Here's how the part is built. I have some questions about the finished solid (model axes, mm). Face numbers are marked on the shaded views. A direction names the side the tool comes from. Round coordinates to 2 decimals unless told otherwise and drop trailing zeros. Loops run counter-clockwise (first coordinate to the right, second up) from the corner with the lowest first, then second, coordinate; pieces in that order, holes last. Notation, with made-up numbers: (54.5, 60) - (99.5, 60) arc R18 ccw to (99.5, 72) - close; hole circle Ø1 at (46, 68.25). An arc over 180 degrees is marked (long way). Return JSON: item names as keys, results as strings. Group by question number.
```python
from build123d import *

# Parameters (mm, degrees)
F0_R     = 2.125
F1_DEPTH = 5
F3_DEPTH = 15
F4_R     = 2.125
F5_DEPTH = 5
F6_R     = 2.125
F7_DEPTH = 5
F9_DEPTH = 5
F10_SIZE = 10


with BuildPart() as f1:
    # F0 (on Top) → F1 (new body)
    with BuildSketch(Plane.XY):
        Polygon((0, 20), (0, 50), (-20, 50), (-20, 0), (30, 0), (30, 20), align=None)
        with Locations((-12.5, 7.5)):
            Circle(F0_R, mode=Mode.SUBTRACT)
        with Locations((20, 7.5)):
            Circle(F0_R, mode=Mode.SUBTRACT)
        with Locations((-12.5, 40)):
            Circle(F0_R, mode=Mode.SUBTRACT)
    extrude(amount=F1_DEPTH)

    # F2 (on face) → F3 (join)
    with BuildSketch(Plane.XY.offset(5)):
        Polygon((0, 20), (0, 50), (-5, 50), (-5, 15), (30, 15), (30, 20), align=None)
    extrude(amount=F3_DEPTH)

    # F4 (on face) → F5 (cut)
    with BuildSketch(Plane(origin=(-5, 0, 0), x_dir=(0, -1, 0), z_dir=(-1, 0, 0))):
        with Locations((-37.5, 12.5)):
            Circle(F4_R)
    extrude(amount=-F5_DEPTH, mode=Mode.SUBTRACT)

    # F6 (on face) → F7 (cut)
    with BuildSketch(Plane.XZ.offset(-15)):
        with Locations((17.5, 12.5)):
            Circle(F6_R)
    extrude(amount=-F7_DEPTH, mode=Mode.SUBTRACT)

    # F8 (on Top) → F9 (join)
    with BuildSketch(Plane.XY):
        Polygon((30, 20), (0, 50), (0, 20), align=None)
    extrude(amount=F9_DEPTH)

    # F10
    f10_edges = [f1.edges().sort_by_distance(p)[0] for p in [
        (0, 20, 12.5),
    ]]
    chamfer(f10_edges, length=F10_SIZE)


solid = f1.part
```
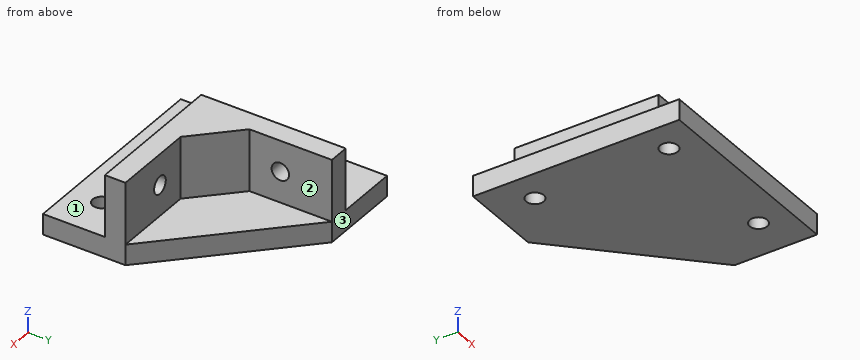
Q1. Imagine slicing it at B-B, the plane z = 12.5. List the corners of the cut face in (x, y) for me (3 decimals), and give its area (4 significant figures).
Q2. Please list where these lines run through material, in increasing order: line 1 (Z direction, x = 17.5, y = 16) (3 decimals); line 2 (Y direction, x = 10, z = 16.5); line 3 (X direction, y = 19.5, z = 19).
Q3. Will these pins go through, and if not, where does the flat tip stop? pin 1 Ø2.5 at (x, y) = (-12.5, 40) entering from -Z; pin 2 Ø1.5 at (x, y) = (-12.5, 33.5) entering from +Z; pin 3 Ø7.5 at (y, z) = (27.5, 15) entering from -X; pin 4 Ø12 at (x, z) = (-1.5, 3) entering from -Y.
Q4. For the marked faces 1, 2 and 3, which set-ups out of +Z, -Z, +X, -X, +Y, -Y let a thin tool reach every point of the face, with its end or its side?
Q5. Imagine slicing it at D-D, the plane z = 18.75. List the corners of the cut face in (x, y) for me.
Q6. Imagine slicing it at C-C, the plane x = -12.5. List the corners of the cut face in (y, z) for me (3 decimals), and give its area (4 significant figures).
Q7. Imagine slicing it at A-A, the plane y = 17.5. List the corners of the cut face in (x, z) for me (3 decimals), and give its area (3 significant figures).
Output values:
{
 "1": {"outline": "(-5, 15) - (15.375, 15) - (15.375, 20) - (10, 20) - (0, 30) - (0, 35.375) - (-5, 35.375) - close; (-5, 39.625) - (0, 39.625) - (0, 50) - (-5, 50) - close; (19.625, 15) - (30, 15) - (30, 20) - (19.625, 20) - close", "area": "332.5 mm^2"},
 "2": {"line 1": "z = 0 to 10.375, 14.625 to 20", "line 2": "y = 15 to 20", "line 3": "x = -5 to 30"},
 "3": {"pin 1": "passes through", "pin 2": "stops at z = 5", "pin 3": "stops at x = -5", "pin 4": "stops at y = 0"},
 "4": {"face 1": "+Z, -X, -Y", "face 2": "+Z, +X, +Y", "face 3": "+Z, -Z, +X, -X, +Y"},
 "5": {"outline": "(-5, 15) - (30, 15) - (30, 20) - (10, 20) - (0, 30) - (0, 50) - (-5, 50) - close"},
 "6": {"outline": "(0, 0) - (5.375, 0) - (5.375, 5) - (0, 5) - close; (9.625, 0) - (37.875, 0) - (37.875, 5) - (9.625, 5) - close; (42.125, 0) - (50, 0) - (50, 5) - (42.125, 5) - close", "area": "207.5 mm^2"},
 "7": {"outline": "(-20, 0) - (30, 0) - (30, 20) - (-5, 20) - (-5, 5) - (-20, 5) - close; hole circle Ø4.25 at (17.5, 12.5)", "area": "761 mm^2"}
}
